Part model, mm, in its own coordinate system. A direction names the side the tool comes from. Round coordinates to 2 decimals unless told otherwise and drop trailing zeros. Write each loop counter-clockwise with the first axis right and the second up, starting at its lowest first coordinate (ties: lowest second). Pieces come first, ordered by that corner, then holes. Notation, with made-up numbers: (56.25, 9) -> (86.25, 9) arc R12 cw to (86.25, 22) -> close; hole circle Ø9 at (56.25, -7.75). An arc over 180 degrees is marked (long way). Use CSV: the item, a comma, the result in double quotes. Start each with the question number.
(1) Which spindle directions (+Z, -Z, +X, -X, +Y, -Y) get a long thin tool onto all of the face, cutting with end or side? Do faces 4 (the cylindrical face through (49, 0, -24)), 5 (the flat face through (-47.213, 11, 0)), 6 (the cylindrical face through (1.1, 11.2, -25.8)). Say none if no direction does.
(2) Probe line 1 (X direction, y = 0.25, z = 6); line 2 (Z direction, x = -27, y = 4.5); line 3 (Y direction, x = 24, z = 22.5). List the from-to ranges inside material, lowest first. Write a range as [from, to].
(3) Drop flat-ended pins along their axis: pin 1 (1.3 mm diameter, centred on x = 14.5, y = -11, fed in from -Z); pin 2 (1.3 mm diameter, centred on y = 11.5, z = -10.5, fed in from -X); pin 3 (0.8 mm diameter, centred on y = -12, z = 0, fed in from -X); pin 4 (6 mm diameter, centred on x = 6.5, y = 8, fed in from +Z). Give the stop position or say it passes through.
(4) Saw through at B-B (x = -9). Give the cut face in (y, z), plus the area to 3 significant figures.
(5) Two-plate mould, pull along Y, no slides. Class faces 1 (the cylindrical face through (49, 0, 24)), 2 (the flat face through (-1, 0, -27.274)), 3 (the cylindrical face through (-1.11, -11.25, 25.75)): released by +Y, released by -Y, zero draft, split by the parting line, or undercut.
(6) Saw through at A-A (z = 2). Give the cut face in (x, y), plus the area to 3 significant figures.
(7) Saw through at C-C (y = 2.75). Give the cut face in (x, z).
```python
from build123d import *

# Parameters (mm, degrees)
F0_W         = 104.5865043998
F0_H         = 54.5481517911
F1_DEPTH     = 12.7
F2_R         = 5.08
F3_T1_DEPTH  = 57.0881517911
F3_T3_DEPTH  = 15.24
F3_T5_DEPTH  = 107.1265043998
F3_S9_W      = 5.1816
F3_S9_H      = 5.1816
F3_T10_DEPTH = 5.1816
F3_S15_W     = 5.1816
F3_S15_H     = 5.1816
F3_T16_DEPTH = 5.1816
F4_T         = -2.54


# Not quite as in the source:
# - a fillet or chamfer that OpenCascade refuses, or shapes differently, is made with other operations: its cross-section is extruded or revolved along the edge and cut away or added
# - a shell that OpenCascade refuses in one call is made with other operations: the cavity is built on its own and cut out


with BuildPart() as f1:
    # F0 (on Front) → F1 (new body, symmetric)
    with BuildSketch(Plane.XZ):
        Rectangle(F0_W, F0_H)
    extrude(amount=F1_DEPTH, both=True)

    # F2
    f2_edges = [f1.edges().sort_by_distance(p)[0] for p in [
        (52.293252, 0, 27.274076),
        (0, 12.7, 27.274076),
        (-52.293252, 0, 27.274076),
        (0, -12.7, 27.274076),
        (52.293252, 0, -27.274076),
        (52.293252, 12.7, 0),
        (52.293252, -12.7, 0),
    ]]
    fillet(f2_edges, radius=F2_R)

    # F3: fillet of radius 5.08 on 7 edges, made by hand

    # F3_s2 → F3_t1 (cut)
    with BuildSketch(Plane.XY.offset(-22.1940758955)):
        with BuildLine():
            ThreePointArc((-47.2132521999, 12.7), (-50.8053546483, 11.2121024484), (-52.2932521999, 7.62))
            Line((-52.2932521999, 7.62), (-52.2932521999, 12.7))
            Line((-52.2932521999, 12.7), (-47.2132521999, 12.7))
        make_face()
        with BuildLine():
            ThreePointArc((-52.2932521999, -7.62), (-50.8053546483, -11.2121024484), (-47.2132521999, -12.7))
            Line((-47.2132521999, -12.7), (-52.2932521999, -12.7))
            Line((-52.2932521999, -12.7), (-52.2932521999, -7.62))
        make_face()
    extrude(amount=F3_T1_DEPTH, mode=Mode.SUBTRACT)

    # F3_s4 → F3_t3 (cut)
    with BuildSketch(Plane.XZ.offset(-7.62)):
        with BuildLine():
            ThreePointArc((-47.2132521999, -27.2740758955), (-50.8053546483, -25.786178344), (-52.2932521999, -22.1940758955))
            Line((-52.2932521999, -22.1940758955), (-52.2932521999, -27.2740758955))
            Line((-52.2932521999, -27.2740758955), (-47.2132521999, -27.2740758955))
        make_face()
    extrude(amount=F3_T3_DEPTH, mode=Mode.SUBTRACT)

    # F3_s6 → F3_t5 (cut)
    with BuildSketch(Plane.YZ.offset(-47.2132521999)):
        with BuildLine():
            ThreePointArc((7.62, -27.2740758955), (11.2121024484, -25.786178344), (12.7, -22.1940758955))
            Line((12.7, -22.1940758955), (12.7, -27.2740758955))
            Line((12.7, -27.2740758955), (7.62, -27.2740758955))
        make_face()
        with BuildLine():
            ThreePointArc((-7.62, -27.2740758955), (-11.2121024484, -25.786178344), (-12.7, -22.1940758955))
            Line((-12.7, -22.1940758955), (-12.7, -27.2740758955))
            Line((-12.7, -27.2740758955), (-7.62, -27.2740758955))
        make_face()
    extrude(amount=F3_T5_DEPTH, mode=Mode.SUBTRACT)


with BuildPart() as f3_tool8:
    # F3_s9 → F3_t10 (new body)
    with BuildSketch(Plane.XY.offset(-22.1940758955)):
        with Locations((-49.8040521999, 10.2108)):
            Rectangle(F3_S9_W, F3_S9_H)
    extrude(amount=-F3_T10_DEPTH)

    # F3_s11 → F3_t12 (revolve, cut)
    with BuildSketch(Plane(origin=(-47.2132521999, 7.62, -22.1940758955), x_dir=(0.7071067812, -0.7071067812, 0), z_dir=(0.7071067812, 0.7071067812, 0))):
        with BuildLine():
            ThreePointArc((0, -5.08), (5.08, 0), (0, 5.08))
            Line((0, 5.08), (0, -5.08))
        make_face()
    revolve(axis=Axis((-47.2132521999, 7.62, -22.1940758955), (0, 0, -1)), mode=Mode.SUBTRACT)


with BuildPart() as f1_1:
    add(f1.part)

    # F3_t7: cut F3_tool8
    add(f3_tool8.part, mode=Mode.SUBTRACT)


with BuildPart() as f3_tool14:
    # F3_s15 → F3_t16 (new body)
    with BuildSketch(Plane.XY.offset(-22.1940758955)):
        with Locations((-49.8040521999, -10.2108)):
            Rectangle(F3_S15_W, F3_S15_H)
    extrude(amount=-F3_T16_DEPTH)

    # F3_s17 → F3_t18 (revolve, cut)
    with BuildSketch(Plane(origin=(-47.2132521999, -7.62, -22.1940758955), x_dir=(0.7071067812, 0.7071067812, 0), z_dir=(-0.7071067812, 0.7071067812, 0))):
        with BuildLine():
            ThreePointArc((0, -5.08), (5.08, 0), (0, 5.08))
            Line((0, 5.08), (0, -5.08))
        make_face()
    revolve(axis=Axis((-47.2132521999, -7.62, -22.1940758955), (0, 0, -1)), mode=Mode.SUBTRACT)


with BuildPart() as f1_2:
    add(f1_1.part)

    # F3_t13: cut F3_tool14
    add(f3_tool14.part, mode=Mode.SUBTRACT)

    # F4: a shell. OpenCascade refuses it in one call, so the cavity is built on its own and cut out:
    # the body offset inwards by the wall thickness, plus a prism from it out through each open face.
    f4_core = offset(f1_2.part, amount=F4_T, mode=Mode.PRIVATE)
    f4_exits = [f4_core.faces().sort_by_distance(p)[0] for p in [
        (0, -10.16, 0),
        (0, 10.16, 0),
    ]]
    add(f4_core, mode=Mode.SUBTRACT)
    extrude(f4_exits, amount=-F4_T, mode=Mode.SUBTRACT)


solid = f1_2.part
```
Answers:
1,face 4,"none"
1,face 5,"+Y, -Y"
1,face 6,"-Z, +X, -X, +Y"
2,line 1,"x = [-52.29, -49.75], [49.75, 52.29]"
2,line 2,"z = [-27.27, -24.73], [24.73, 27.27]"
2,line 3,"y = [-12.69, -10.14], [10.14, 12.69]"
3,pin 1,"stops at z = -26.48"
3,pin 2,"stops at x = -51.13"
3,pin 3,"stops at x = -50.37"
3,pin 4,"stops at z = 27.27"
4,outline,"(-12.7, -22.19) arc R5.08 ccw to (-7.62, -27.27) -> (7.62, -27.27) arc R5.08 ccw to (12.7, -22.19) -> (10.16, -22.19) arc R2.54 cw to (7.62, -24.73) -> (-7.62, -24.73) arc R2.54 cw to (-10.16, -22.19) -> close; (-12.7, 22.19) -> (-10.16, 22.19) arc R2.54 cw to (-7.62, 24.73) -> (7.62, 24.73) arc R2.54 cw to (10.16, 22.19) -> (12.7, 22.19) arc R5.08 ccw to (7.62, 27.27) -> (-7.62, 27.27) arc R5.08 ccw to start"
4,area,"138 mm²"
5,face 1,"undercut"
5,face 2,"zero draft"
5,face 3,"released by -Y"
6,outline,"(-52.29, -7.62) arc R5.08 ccw to (-47.21, -12.7) -> (-47.21, -10.16) arc R2.54 cw to (-49.75, -7.62) -> (-49.75, 7.62) arc R2.54 cw to (-47.21, 10.16) -> (-47.21, 12.7) arc R5.08 ccw to (-52.29, 7.62) -> close; (47.21, -12.7) arc R5.08 ccw to (52.29, -7.62) -> (52.29, 7.62) arc R5.08 ccw to (47.21, 12.7) -> (47.21, 10.16) arc R2.54 cw to (49.75, 7.62) -> (49.75, -7.62) arc R2.54 cw to (47.21, -10.16) -> close"
6,area,"138 mm²"
7,outline,"(-52.29, -22.19) arc R5.08 ccw to (-47.21, -27.27) -> (47.21, -27.27) arc R5.08 ccw to (52.29, -22.19) -> (52.29, 22.19) arc R5.08 ccw to (47.21, 27.27) -> (-47.21, 27.27) arc R5.08 ccw to (-52.29, 22.19) -> close; hole (-49.75, -22.19) arc R2.54 ccw to (-47.21, -24.73) -> (47.21, -24.73) arc R2.54 ccw to (49.75, -22.19) -> (49.75, 22.19) arc R2.54 ccw to (47.21, 24.73) -> (-47.21, 24.73) arc R2.54 ccw to (-49.75, 22.19) -> close"
